```python
from build123d import *

# Parameters (mm, degrees)
SKETCH_1_R          = 1.3
SKETCH_1_R_2        = 5
SKETCH_1_R_3        = 1.45
EXTRUDE_1_DEPTH     = 2
SKETCH_2_R          = 3
CUT_EXTRUDE_1_DEPTH = 0.8
SKETCH_4_W          = 8.73447759
SKETCH_4_H          = 10.120774017
CUT_EXTRUDE_2_DEPTH = 33.667542419
SKETCH_8_R          = 2.25
SKETCH_8_R_2        = 1.45
EXTRUDE_2_DEPTH     = 2
CUT_EXTRUDE_4_DEPTH = 1
FILLET_3_R          = 3


with BuildPart() as part:
    # 草图1 → 凸台-拉伸1 (new body)
    with BuildSketch(Plane(origin=(0, 0, 0), x_dir=(1, 0, 0), z_dir=(0, 1, 0))):
        with BuildLine():
            Line((-19.570385791, 15.556349186), (-19.570385791, -15.556349186))
            Line((-19.570385791, -15.556349186), (-19.570385791, -17.556349186))
            ThreePointArc((-19.570385791, -17.556349186), (-10.696991496, -23.91128764), (0, -26.07848445))
            ThreePointArc((0, -26.07848445), (10.696991496, -23.91128764), (19.570385791, -17.556349186))
            Line((19.570385791, -17.556349186), (19.570385791, -15.556349186))
            Line((19.570385791, -15.556349186), (19.570385791, 15.556349186))
            Line((19.570385791, 15.556349186), (19.570385791, 17.556349186))
            ThreePointArc((19.570385791, 17.556349186), (10.696991496, 23.91128764), (0, 26.07848445))
            ThreePointArc((0, 26.07848445), (-10.696991496, 23.91128764), (-19.570385791, 17.556349186))
            Line((-19.570385791, 17.556349186), (-19.570385791, 15.556349186))
        make_face()
        with Locations(Location((0, 9, 0), (0, 0, 270))):
            Circle(SKETCH_1_R, mode=Mode.SUBTRACT)
        with Locations(Location((7.794228634, -4.5, 0), (0, 0, 270))):
            Circle(SKETCH_1_R, mode=Mode.SUBTRACT)
        with Locations(Location((-7.794228634, -4.5, 0), (0, 0, 270))):
            Circle(SKETCH_1_R, mode=Mode.SUBTRACT)
        with Locations(Location((0, 0, 0), (0, 0, 270))):
            Circle(SKETCH_1_R_2, mode=Mode.SUBTRACT)
        with Locations(Location((-15.556349186, 15.556349186, 0), (0, 0, 270))):
            Circle(SKETCH_1_R_3, mode=Mode.SUBTRACT)
        with Locations(Location((15.556349186, 15.556349186, 0), (0, 0, 270))):
            Circle(SKETCH_1_R_3, mode=Mode.SUBTRACT)
        with Locations(Location((15.556349186, -15.556349186, 0), (0, 0, 270))):
            Circle(SKETCH_1_R_3, mode=Mode.SUBTRACT)
        with Locations(Location((-15.556349186, -15.556349186, 0), (0, 0, 270))):
            Circle(SKETCH_1_R_3, mode=Mode.SUBTRACT)
    extrude(amount=EXTRUDE_1_DEPTH)

    # 草图2 → 切除-拉伸1 (cut)
    with BuildSketch(Plane(origin=(0, 2, 0), x_dir=(1, 0, 0), z_dir=(0, 1, 0))):
        with Locations(Location((0, 9, 0), (0, 0, 270))):
            Circle(SKETCH_2_R)
        with Locations(Location((7.794228634, -4.5, 0), (0, 0, 270))):
            Circle(SKETCH_2_R)
        with Locations(Location((-7.794228634, -4.5, 0), (0, 0, 270))):
            Circle(SKETCH_2_R)
    extrude(amount=-CUT_EXTRUDE_1_DEPTH, mode=Mode.SUBTRACT)

    # 草图4 → 切除-拉伸2 (cut, through all)
    with BuildSketch(Plane(origin=(0, 2, 0), x_dir=(1, 0, 0), z_dir=(0, 1, 0))):
        Polygon((-3.274193367, -19.855122702), (-3.274193367, -7.205990029), (3.274193367, -7.205990029), (3.274193367, -19.855122702), (19.611727687, -19.855122702), (19.611727687, -26.506793376), (-19.611727687, -26.506793376), (-19.611727687, -19.855122702), align=None)
        with Locations((0, 21.431925769)):
            Rectangle(SKETCH_4_W, SKETCH_4_H)
    extrude(amount=-CUT_EXTRUDE_2_DEPTH, mode=Mode.SUBTRACT)

    # 草图8 → 凸台-拉伸2 (add)
    # profile 1 of 4: a face of its own
    with BuildSketch(Plane(origin=(0, 2, 0), x_dir=(1, 0, 0), z_dir=(0, 1, 0))):
        with Locations(Location((-15.556349186, 15.556349186, 0), (0, 0, 270))):
            Circle(SKETCH_8_R)
        with Locations(Location((-15.556349186, 15.556349186, 0), (0, 0, 270))):
            Circle(SKETCH_8_R_2, mode=Mode.SUBTRACT)
    # profile 2 of 4: a face of its own
    with BuildSketch(Plane(origin=(0, 2, 0), x_dir=(1, 0, 0), z_dir=(0, 1, 0))):
        with Locations(Location((15.556349186, 15.556349186, 0), (0, 0, 270))):
            Circle(SKETCH_8_R)
        with Locations(Location((15.556349186, 15.556349186, 0), (0, 0, 270))):
            Circle(SKETCH_8_R_2, mode=Mode.SUBTRACT)
    # profile 3 of 4: a face of its own
    with BuildSketch(Plane(origin=(0, 2, 0), x_dir=(1, 0, 0), z_dir=(0, 1, 0))):
        with Locations(Location((15.556349186, -15.556349186, 0), (0, 0, 270))):
            Circle(SKETCH_8_R)
        with Locations(Location((15.556349186, -15.556349186, 0), (0, 0, 270))):
            Circle(SKETCH_8_R_2, mode=Mode.SUBTRACT)
    # profile 4 of 4: a face of its own
    with BuildSketch(Plane(origin=(0, 2, 0), x_dir=(1, 0, 0), z_dir=(0, 1, 0))):
        with Locations(Location((-15.556349186, -15.556349186, 0), (0, 0, 270))):
            Circle(SKETCH_8_R)
        with Locations(Location((-15.556349186, -15.556349186, 0), (0, 0, 270))):
            Circle(SKETCH_8_R_2, mode=Mode.SUBTRACT)
    extrude(amount=EXTRUDE_2_DEPTH)

    # 草图7 → 切除-拉伸4 (cut)
    with BuildSketch(Plane.XZ):
        Polygon((-18.732353017, 15.556349186), (-17.144351102, 12.805849186), (-13.968347271, 12.805849186), (-12.380345355, 15.556349186), (-13.968347271, 18.306849186), (-17.144351102, 18.306849186), align=None)
        Polygon((12.380345355, 15.556349186), (13.968347271, 12.805849186), (17.144351102, 12.805849186), (18.732353017, 15.556349186), (17.144351102, 18.306849186), (13.968347271, 18.306849186), align=None)
        Polygon((-18.732353017, -15.556349186), (-17.144351102, -18.306849186), (-13.968347271, -18.306849186), (-12.380345355, -15.556349186), (-13.968347271, -12.805849186), (-17.144351102, -12.805849186), align=None)
        Polygon((12.380345355, -15.556349186), (13.968347271, -18.306849186), (17.144351102, -18.306849186), (18.732353017, -15.556349186), (17.144351102, -12.805849186), (13.968347271, -12.805849186), align=None)
    extrude(amount=-CUT_EXTRUDE_4_DEPTH, mode=Mode.SUBTRACT)

    # 圆角3
    fillet_3_edges = [part.edges().sort_by_distance(p)[0] for p in [
        (3.274193367, 1, 19.855122702),
        (-3.274193367, 1, 7.205990029),
        (3.274193367, 1, 7.205990029),
        (-3.274193367, 1, 19.855122702),
        (19.570385791, 1, -17.556349186),
        (-19.570385791, 1, -17.556349186),
        (-4.367238795, 1, -25.758495538),
        (4.367238795, 1, -25.758495538),
    ]]
    fillet(fillet_3_edges, radius=FILLET_3_R)


solid = part.part
```
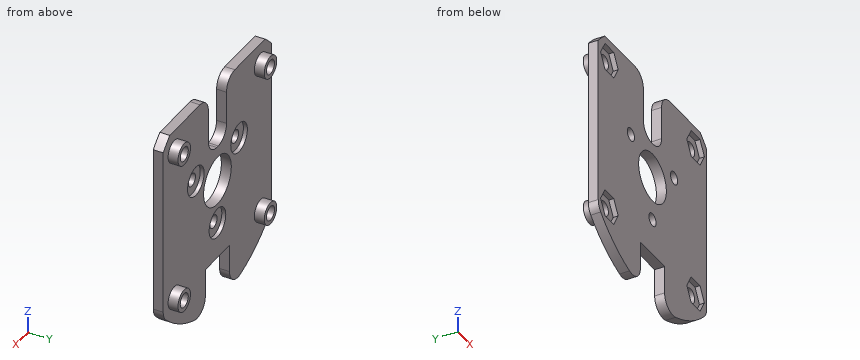
Check sheet for the modelled part. Datum: model origin and axes. Units: mm. Coordinates: 2 decimals unless noted, no trailing zeros. Loops run counter-clockwise (first coordinate to the right, second up) from the corner with the lowest first, then second, coordinate; pieces in that order, holes last.
1) Gauge pin test, flat ends, axial feed: pin 1 (1 mm diameter, centred on y = 1, z = -19.5, fed in from +X); pin 2 (3 mm diameter, centred on x = -0.5, z = -8, fed in from +Y); pin 3 (0.8 mm diameter, centred on x = -16.5, y = 0.5, fed in from -Z); pin 4 (2 mm diameter, centred on x = -7.79, z = 4.5, fed in from +Y). Record the tip position at first contact, or that the pin passes through.
2) Sectioned sample at C-C (z = 4.5). Record the boundary of the cut face in (x, y), and give its area (3 significant figures).
3) Sectioned sample at B-B (z = 0). Record the boundary of the cut face in (x, y).
4) Sectioned sample at D-D (x = -5.5). Record the boundary of the cut face in (y, z), and give its area (3 significant figures).
5) Sectioned sample at A-A (y = 2.8). Record the boundary of the cut face in (x, z), and give its area (3 significant figures).
6) Material ranges on probe 1 along X at (y, z) = (1.35, 0); probe 2 along Z at (x, y) = (15.5, 1.35); probe 3 along X at (y, z) = (1.3, -14.5), recorded low to high.
Check sheet entries:
1. pin 1: stops at x = 18.15
1. pin 2: stops at y = 1.2
1. pin 3: stops at z = -20.74
1. pin 4: passes through
2. outline: (-19.57, 0) - (-9.09, 0) - (-9.09, 1.2) - (-10.79, 1.2) - (-10.79, 2) - (-19.57, 2) - close; (-6.49, 0) - (-2.18, 0) - (-2.18, 2) - (-4.79, 2) - (-4.79, 1.2) - (-6.49, 1.2) - close; (2.18, 0) - (6.49, 0) - (6.49, 1.2) - (4.79, 1.2) - (4.79, 2) - (2.18, 2) - close; (9.09, 0) - (19.57, 0) - (19.57, 2) - (10.79, 2) - (10.79, 1.2) - (9.09, 1.2) - close
2. area: 53.7 mm2
3. outline: (-19.57, 0) - (-5, 0) - (-5, 2) - (-19.57, 2) - close; (5, 0) - (19.57, 0) - (19.57, 2) - (5, 2) - close
4. outline: (0, -24.31) - (2, -24.31) - (2, 2.57) - (1.2, 2.57) - (1.2, 6.43) - (2, 6.43) - (2, 19.75) - (0, 19.75) - close
4. area: 85.0 mm2
5. outline: circle Ø4.5 at (-15.56, -15.56); circle Ø4.5 at (-15.56, 15.56); circle Ø4.5 at (15.56, -15.56); circle Ø4.5 at (15.56, 15.56); hole circle Ø2.9 at (-15.56, -15.56); hole circle Ø2.9 at (-15.56, 15.56); hole circle Ø2.9 at (15.56, -15.56); hole circle Ø2.9 at (15.56, 15.56)
5. area: 37.2 mm2
6. probe 1: x = -19.57 to -5, 5 to 19.57
6. probe 2: z = -21.18 to -17.01, -14.11 to 14.11, 17.01 to 19.86
6. probe 3: x = -19.57 to -16.55, -14.56 to 14.56, 16.55 to 19.57
